Part model, mm, in its own coordinate system. Face numbers are marked on the shaded views. Coordinates: 2 decimals unless noted, no trailing zeros. Loops run counter-clockwise (first coordinate to the right, second up) from the corner with the lowest first, then second, coordinate; pieces in that order, holes last. Notation, with made-up numbers: (-1.75, -31.75) - (8.25, -31.75) arc R21 ccw to (8.25, -23.75) - close; hole circle Ø4 at (-39, -24.75). An arc over 180 degrees is marked (long way). Use a Markdown table: item, result. Add a question column.
1) Drop a flat-ended pin along its axis: P1, Ø5, axis at x = 64.5, z = -32.5, coming from the -Y side. Give the stop position or say it passes through.
2) Pull direction X, two halves, no side cores. Call the marked faces 1, 2, 3 and 4: +X half, -X half, draft (parallel to the pull), parting line (faces both ways), or undercut.
3) Probe probe 1 along X at (y, z) = (-98.5, -44); probe 2 along Z at (x, y) = (60, -36); probe 3 along Y at (x, z) = (-42.5, 31). List the from-to ranges inside material, lowest first. Write a range as [from, to].
4) Band-saw the part on A-A (y = -105.5). Give the cut face in (x, z).
5) Band-saw the part on B-B (x = 49). Give the cut face in (y, z), plus the area to 3 significant figures.
6) Band-saw the part on C-C (z = -37). Give the cut face in (x, y).
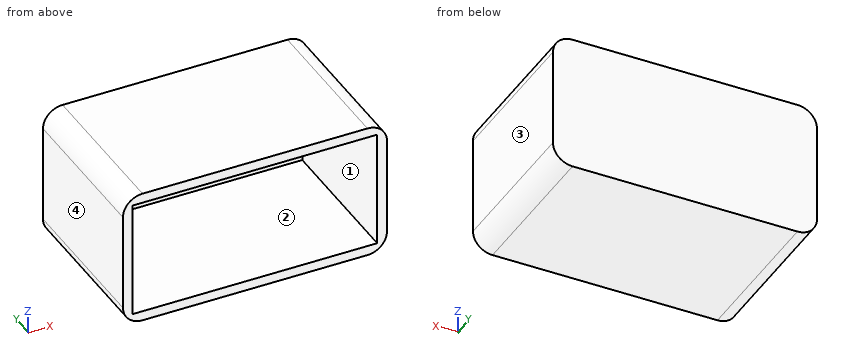
from build123d import *

# Parameters (mm, degrees)
F0_W     = 270
F0_H     = 140
F1_DEPTH = 160
F2_T     = -10
F3_R     = 20


with BuildPart() as f1:
    # F0 (on Front) → F1 (new body)
    with BuildSketch(Plane.XZ):
        Rectangle(F0_W, F0_H)
    extrude(amount=F1_DEPTH)

    # F2
    f2_openings = [f1.faces().sort_by_distance(p)[0] for p in [
        (0, -160, 0),
    ]]
    offset(amount=F2_T, openings=f2_openings)

    # F3
    f3_edges = [f1.edges().sort_by_distance(p)[0] for p in [
        (-135, -80, 70),
        (135, -80, -70),
        (135, -80, 70),
        (-135, -80, -70),
    ]]
    fillet(f3_edges, radius=F3_R)


solid = f1.part
Answer block:
| question | item | result |
|---|---|---|
| 1 | P1 | y = -10 |
| 2 | face 1 | undercut |
| 2 | face 2 | undercut |
| 2 | face 3 | +X half |
| 2 | face 4 | -X half |
| 3 | probe 1 | [-135, -125], [125, 135] |
| 3 | probe 2 | [-70, -60], [60, 70] |
| 3 | probe 3 | [-10, 0] |
| 4 | outline | (-135, -50) arc R20 ccw to (-115, -70) - (115, -70) arc R20 ccw to (135, -50) - (135, 50) arc R20 ccw to (115, 70) - (-115, 70) arc R20 ccw to (-135, 50) - close; hole (-125, -60) - (125, -60) - (125, 60) - (-125, 60) - close |
| 5 | outline | (-160, -70) - (0, -70) - (0, 70) - (-160, 70) - (-160, 60) - (-10, 60) - (-10, -60) - (-160, -60) - close |
| 5 | area | 4,400 mm2 |
| 6 | outline | (-135, -160) - (-125, -160) - (-125, -10) - (125, -10) - (125, -160) - (135, -160) - (135, 0) - (-135, 0) - close |
